Check sheet for the drawn part. Datum: minimum x, y, z corner. Units: mm. Give positions to 0.01 mm unless a question says otherwise; leave off trailing zeros. Loops run counter-clockwise (first coordinate to the right, second up) from the corner with the lowest first, then second, coordinate; pieces in that order, holes last. Notation, with made-up numbers: M 10.5,63 L 32.5,63 A22 cw 32.5,93 Z; hole C -11.75,-31 d11. An arc over 180 degrees is marked long. Write each question's results on one line, items separated by ' | '. Start each with the question number.
1. Material ranges on line 1 along X through (y, z) = (4.75, 7.25); line 2 along X through (y, z) = (3.75, 1.25); line 3 along Y through (x, z) = (27.5, 4), recorded low to high.
2. Sectioned sample at B-B on x = 27.5. Record the cut outline in (y, z).
3. Draft check along Y on the marked faces 1, 2 and 3. Enter one of: pulls with the +Y half, pulls with the -Y half, needs draft (parallel to the pull), parting line crosses it, or undercut.
4. Sectioned sample at D-D on y = 7. Record the cut outline in (x, z).
5. Sectioned sample at C-C on z = 1. Record the cut outline in (x, y) (3 decimals), and give its area (3 significant figures).
6. Sectioned sample at A-A on y = 5. Record the cut outline in (x, z).
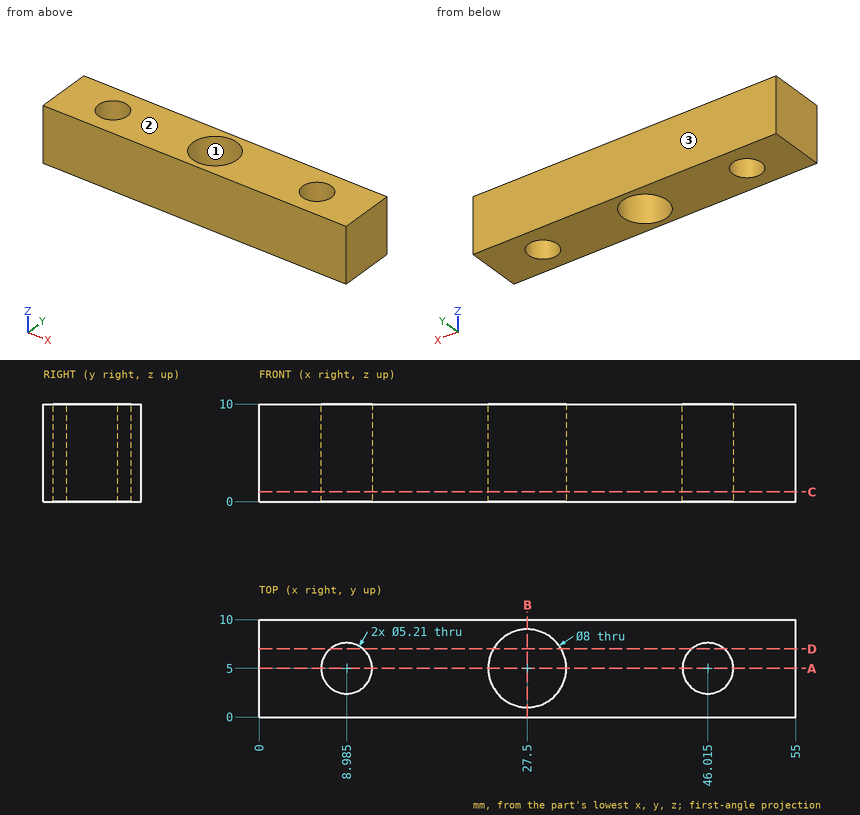
Output values:
1) line 1: 0 to 6.39, 11.58 to 23.51, 31.49 to 43.42, 48.61 to 55 | line 2: 0 to 6.7, 11.27 to 23.7, 31.3 to 43.73, 48.3 to 55 | line 3: 0 to 1, 9 to 10
2) outline: M 0,0 L 1,0 L 1,10 L 0,10 Z; M 9,0 L 10,0 L 10,10 L 9,10 Z
3) face 1: undercut | face 2: needs draft | face 3: pulls with the +Y half
4) outline: M 0,0 L 7.32,0 L 7.32,10 L 0,10 Z; M 10.65,0 L 24.04,0 L 24.04,10 L 10.65,10 Z; M 30.96,0 L 44.35,0 L 44.35,10 L 30.96,10 Z; M 47.68,0 L 55,0 L 55,10 L 47.68,10 Z
5) outline: M 0,0 L 55,0 L 55,10 L 0,10 Z; hole C 8.985,5 d5.21; hole C 27.5,5 d8; hole C 46.015,5 d5.21 | area: 457 mm2
6) outline: M 0,0 L 6.38,0 L 6.38,10 L 0,10 Z; M 11.59,0 L 23.5,0 L 23.5,10 L 11.59,10 Z; M 31.5,0 L 43.41,0 L 43.41,10 L 31.5,10 Z; M 48.62,0 L 55,0 L 55,10 L 48.62,10 Z
